from build123d import *

# Parameters (mm, degrees)
SKETCH1_W                    = 295.275
SKETCH1_H                    = 174.625
BASE_FLANGE1_DEPTH           = 3.175
EDGE_FLANGE1_STRIP_W         = 14.1732
EDGE_FLANGE1_STRIP_H         = 3.175
EDGE_FLANGE1_STRIP_CUT_DEPTH = 174.625
EDGE_FLANGE1_DEPTH           = 174.625
EDGE_FLANGE2_STRIP_W         = 14.1732
EDGE_FLANGE2_STRIP_H         = 3.175
EDGE_FLANGE2_STRIP_CUT_DEPTH = 307.2384
EDGE_FLANGE2_DEPTH           = 307.2384
EDGE_FLANGE3_STRIP_W         = 14.1732
EDGE_FLANGE3_STRIP_H         = 3.175
EDGE_FLANGE3_STRIP_CUT_DEPTH = 307.2384
EDGE_FLANGE3_DEPTH           = 307.2384
EDGE_FLANGE4_STRIP_W         = 14.1732
EDGE_FLANGE4_STRIP_H         = 3.175
EDGE_FLANGE4_STRIP_CUT_DEPTH = 166.8018
EDGE_FLANGE4_DEPTH           = 166.8018
EDGE_FLANGE5_STRIP_W         = 14.1732
EDGE_FLANGE5_STRIP_H         = 3.175
EDGE_FLANGE5_STRIP_CUT_DEPTH = 174.625
EDGE_FLANGE5_DEPTH           = 174.625
CUT_EXTRUDE1_REACH           = 437.499
EDGE_FLANGE7_STRIP_W         = 14.1732
EDGE_FLANGE7_STRIP_H         = 3.175
EDGE_FLANGE7_STRIP_CUT_DEPTH = 78.994
EDGE_FLANGE7_DEPTH           = 78.994


# Sheet-metal steps are written as plain solids
with BuildPart() as part:
    # Sketch1 → Base-Flange1 (new body)
    with BuildSketch(Plane(origin=(0, 0, 0), x_dir=(1, 0, 0), z_dir=(0, 1, 0))):
        Rectangle(SKETCH1_W, SKETCH1_H)
    extrude(amount=-BASE_FLANGE1_DEPTH)

    # Edge-Flange1 strip (across the edge) → Edge-Flange1 strip cut (cut)
    with BuildSketch(Plane(origin=(-147.6375, 0, -87.3125), x_dir=(1, 0, 0), z_dir=(0, 0, 1))):
        with Locations((-3.175, -1.5875)):
            Rectangle(EDGE_FLANGE1_STRIP_W, EDGE_FLANGE1_STRIP_H)
    extrude(amount=EDGE_FLANGE1_STRIP_CUT_DEPTH, mode=Mode.SUBTRACT)

    # Edge-Flange1 section (across the edge) → Edge-Flange1 (add)
    with BuildSketch(Plane(origin=(-147.6375, 0, -87.3125), x_dir=(1, 0, 0), z_dir=(0, 0, 1))):
        with BuildLine():
            Line((0, 0.7366), (0, 307.975))
            Line((0, 307.975), (3.175, 307.975))
            Line((3.175, 307.975), (3.175, 0.7366))
            ThreePointArc((3.175, 0.7366), (3.390745145, 0.215745145), (3.9116, 0))
            Line((3.9116, 0), (3.9116, -3.175))
            ThreePointArc((3.9116, -3.175), (1.145681115, -2.029318885), (0, 0.7366))
        make_face()
    extrude(amount=EDGE_FLANGE1_DEPTH)

    # Edge-Flange2 strip (across the edge) → Edge-Flange2 strip cut (cut)
    with BuildSketch(Plane(origin=(-144.4625, 307.975, 87.3125), x_dir=(0, 0, -1), z_dir=(0, -1, 0))):
        with Locations((-3.175, -1.5875)):
            Rectangle(EDGE_FLANGE2_STRIP_W, EDGE_FLANGE2_STRIP_H)
    extrude(amount=EDGE_FLANGE2_STRIP_CUT_DEPTH, mode=Mode.SUBTRACT)

    # Edge-Flange2 section (across the edge) → Edge-Flange2 (add)
    with BuildSketch(Plane(origin=(-144.4625, 307.975, 87.3125), x_dir=(0, 0, -1), z_dir=(0, -1, 0))):
        with BuildLine():
            Line((0, 0.7366), (0, 37.465))
            Line((0, 37.465), (3.175, 37.465))
            Line((3.175, 37.465), (3.175, 0.7366))
            ThreePointArc((3.175, 0.7366), (3.390745145, 0.215745145), (3.9116, 0))
            Line((3.9116, 0), (3.9116, -3.175))
            ThreePointArc((3.9116, -3.175), (1.145681115, -2.029318885), (0, 0.7366))
        make_face()
    extrude(amount=EDGE_FLANGE2_DEPTH)

    # Edge-Flange3 strip (across the edge) → Edge-Flange3 strip cut (cut)
    with BuildSketch(Plane(origin=(-144.4625, 0.7366, -87.3125), x_dir=(0, 0, 1), z_dir=(0, 1, 0))):
        with Locations((-3.175, -1.5875)):
            Rectangle(EDGE_FLANGE3_STRIP_W, EDGE_FLANGE3_STRIP_H)
    extrude(amount=EDGE_FLANGE3_STRIP_CUT_DEPTH, mode=Mode.SUBTRACT)

    # Edge-Flange3 section (across the edge) → Edge-Flange3 (add)
    with BuildSketch(Plane(origin=(-144.4625, 0.7366, -87.3125), x_dir=(0, 0, 1), z_dir=(0, 1, 0))):
        with BuildLine():
            Line((0, 0.7366), (0, 37.465))
            Line((0, 37.465), (3.175, 37.465))
            Line((3.175, 37.465), (3.175, 0.7366))
            ThreePointArc((3.175, 0.7366), (3.390745145, 0.215745145), (3.9116, 0))
            Line((3.9116, 0), (3.9116, -3.175))
            ThreePointArc((3.9116, -3.175), (1.145681115, -2.029318885), (0, 0.7366))
        make_face()
    extrude(amount=EDGE_FLANGE3_DEPTH)

    # Edge-Flange4 strip (across the edge) → Edge-Flange4 strip cut (cut)
    with BuildSketch(Plane(origin=(-144.4625, 307.975, -83.4009), x_dir=(0, -1, 0), z_dir=(0, 0, 1))):
        with Locations((-3.175, -1.5875)):
            Rectangle(EDGE_FLANGE4_STRIP_W, EDGE_FLANGE4_STRIP_H)
    extrude(amount=EDGE_FLANGE4_STRIP_CUT_DEPTH, mode=Mode.SUBTRACT)

    # Edge-Flange4 section (across the edge) → Edge-Flange4 (add)
    with BuildSketch(Plane(origin=(-144.4625, 307.975, -83.4009), x_dir=(0, -1, 0), z_dir=(0, 0, 1))):
        with BuildLine():
            Line((0, 0.7366), (0, 37.465))
            Line((0, 37.465), (3.175, 37.465))
            Line((3.175, 37.465), (3.175, 0.7366))
            ThreePointArc((3.175, 0.7366), (3.390745145, 0.215745145), (3.9116, 0))
            Line((3.9116, 0), (3.9116, -3.175))
            ThreePointArc((3.9116, -3.175), (1.145681115, -2.029318885), (0, 0.7366))
        make_face()
    extrude(amount=EDGE_FLANGE4_DEPTH)

    # Edge-Flange5 strip (across the edge) → Edge-Flange5 strip cut (cut)
    with BuildSketch(Plane(origin=(147.6375, 0, 87.3125), x_dir=(-1, 0, 0), z_dir=(0, 0, -1))):
        with Locations((-3.175, -1.5875)):
            Rectangle(EDGE_FLANGE5_STRIP_W, EDGE_FLANGE5_STRIP_H)
    extrude(amount=EDGE_FLANGE5_STRIP_CUT_DEPTH, mode=Mode.SUBTRACT)

    # Edge-Flange5 section (across the edge) → Edge-Flange5 (add)
    with BuildSketch(Plane(origin=(147.6375, 0, 87.3125), x_dir=(-1, 0, 0), z_dir=(0, 0, -1))):
        with BuildLine():
            Line((0, 0.7366), (0, 307.975))
            Line((0, 307.975), (3.175, 307.975))
            Line((3.175, 307.975), (3.175, 0.7366))
            ThreePointArc((3.175, 0.7366), (3.390745145, 0.215745145), (3.9116, 0))
            Line((3.9116, 0), (3.9116, -3.175))
            ThreePointArc((3.9116, -3.175), (1.145681115, -2.029318885), (0, 0.7366))
        make_face()
    extrude(amount=EDGE_FLANGE5_DEPTH)

    # Sketch29 → Cut-Extrude1 (cut, up to next)
    with BuildSketch(Plane(origin=(147.6375, 0, 0), x_dir=(0, 0, -1), z_dir=(1, 0, 0)), mode=Mode.PRIVATE) as cut_extrude1_sk1:
        Polygon((-87.3125, 37.8968), (-68.5673, 56.642), (-12.3825, 56.642), (8.3185, 77.343), (8.3185, 307.975), (-87.3125, 307.975), align=None)
    cut_extrude1_tool1 = extrude(cut_extrude1_sk1.sketch, amount=-CUT_EXTRUDE1_REACH, mode=Mode.PRIVATE) & part.part
    add(cut_extrude1_tool1.solids().sort_by_distance((147.6375, 182.403147, 40.166664))[0], mode=Mode.SUBTRACT)

    # Edge-Flange7 strip (across the edge) → Edge-Flange7 strip cut (cut)
    with BuildSketch(Plane(origin=(144.4625, 307.975, -8.3185), x_dir=(0, -1, 0), z_dir=(0, 0, -1))):
        with Locations((-3.175, -1.5875)):
            Rectangle(EDGE_FLANGE7_STRIP_W, EDGE_FLANGE7_STRIP_H)
    extrude(amount=EDGE_FLANGE7_STRIP_CUT_DEPTH, mode=Mode.SUBTRACT)

    # Edge-Flange7 section (across the edge) → Edge-Flange7 (add)
    with BuildSketch(Plane(origin=(144.4625, 307.975, -8.3185), x_dir=(0, -1, 0), z_dir=(0, 0, -1))):
        with BuildLine():
            Line((0, 0.7366), (0, 250.19))
            Line((0, 250.19), (3.175, 250.19))
            Line((3.175, 250.19), (3.175, 0.7366))
            ThreePointArc((3.175, 0.7366), (3.390745145, 0.215745145), (3.9116, 0))
            Line((3.9116, 0), (3.9116, -3.175))
            ThreePointArc((3.9116, -3.175), (1.145681115, -2.029318885), (0, 0.7366))
        make_face()
    extrude(amount=EDGE_FLANGE7_DEPTH)


solid = part.part
The listing builds one solid part. Answer for the finished solid, in the listing's coordinates (mm). A direction names the side the tool comes from. Coordinates: 2 decimals unless noted, no trailing zeros. Order: outer loops, then holes, each group sorted by start corner. A loop starts at its lowest first (then second) coordinate and runs counter-clockwise, first axis right, second up. Notation, with made-up numbers: (46.25, 45) -> (61.25, 45) arc R28 ccw to (61.25, 68) -> close; hole circle Ø4 at (72.25, 64). An arc over 180 degrees is marked (long way). Answer in a Markdown table with one row per item. Add a question column.
Item 1: Which of the six approach directions +Z, -Z, +X, -X, +Y, -Y give full straight-line access (tool end or side, diameter ignored) to faces 5 (the face through (-144.462, 155, -1)), 6 (the face through (-2, 0, -1)), 7 (the face through (146.07, 47.14, 78.07))?
Item 2: Find section A-A (x = -50). Write down the section's boundary in (y, z) (1 decimal).
Item 3: Find section B-B (x = -111.5). Write down the section's boundary in (y, z) (1 decimal), then the cut area to 4 significant figures.
Item 4: Find section D-D (z = -30). Write down the section's boundary in (x, y) (1 decimal), then the cut area to 3 significant figures.
Item 5: Determine the mould class of faces 1 (the face through (-2, -3.175, -1)), 2 (the face through (-125, 152, -84.138)), 3 (the face through (17, 304.8, -47)), 4 (the face through (-126, 307.975, -1)) for opening direction Y: +Y half, -Y half, draft (parallel to the pull), parting line (faces both ways), or undercut.
Item 6: Find the intervals of material crossed by L1, parallel to X at y = 79, z = -60; L2, parallel to Y at x = -130, z = -36.5 (3 decimals); L3, parallel to X at y = 264, z = 67, in increasing order. Write a range as from..to.
Item 7: Each of these flat-tipped pins is pushed along its axis until it touches: P1, Ø3.5, axis at y = 306.5, z = -38, coming from the -X side; P2, Ø1, axis at x = -145.5, y = 305.5, coming from the +Z side; P3, Ø10, axis at y = 276.5, z = 53, coming from the +X side. Where does it stop, or does it pass through?
Item 8: Find section C-C (y = 281.5). Write down the section's boundary in (x, z), then the cut area to 3 significant figures.
Result set:
| question | item | result |
|---|---|---|
| 1 | face 5 | none |
| 1 | face 6 | +Z, -Z |
| 1 | face 7 | +Z, +X, +Y |
| 2 | outline | (-3.2, -87.3) -> (0, -87.3) -> (0, 87.3) -> (-3.2, 87.3) -> close; (304.8, -87.3) -> (308, -87.3) -> (308, -8.3) -> (304.8, -8.3) -> close |
| 3 | outline | (-3.2, -87.3) -> (0, -87.3) -> (0, 87.3) -> (-3.2, 87.3) -> close; (0.7, -87.3) -> (308, -87.3) -> (308, -84.1) -> (0.7, -84.1) -> close; (0.7, 84.1) -> (308, 84.1) -> (308, 87.3) -> (0.7, 87.3) -> close; (304.8, -83.4) -> (308, -83.4) -> (308, 83.4) -> (304.8, 83.4) -> close |
| 3 | area | 3,035 mm² |
| 4 | outline | (-147.6, 0.7) arc R3.9 ccw to (-143.7, -3.2) -> (143.7, -3.2) arc R3.9 ccw to (147.6, 0.7) -> (147.6, 304.1) arc R3.9 ccw to (143.7, 308) -> (-105.7, 308) -> (-105.7, 304.8) -> (143.7, 304.8) arc R0.7 cw to (144.5, 304.1) -> (144.5, 0.7) arc R0.7 cw to (143.7, 0) -> (-143.7, 0) arc R0.7 cw to (-144.5, 0.7) -> (-144.5, 304.1) arc R0.7 cw to (-143.7, 304.8) -> (-107, 304.8) -> (-107, 308) -> (-143.7, 308) arc R3.9 ccw to (-147.6, 304.1) -> close |
| 4 | area | 3,790 mm² |
| 5 | face 1 | -Y half |
| 5 | face 2 | draft |
| 5 | face 3 | undercut |
| 5 | face 4 | +Y half |
| 6 | L1 | x = -147.64..-144.46, 144.46..147.64 |
| 6 | L2 | y = -3.175..0, 304.8..307.975 |
| 6 | L3 | x = -147.64..-144.46 |
| 7 | P1 | stops at x = -147.58 |
| 7 | P2 | stops at z = 87.1 |
| 7 | P3 | stops at x = -144.46 |
| 8 | outline | (-147.64, -83.4) arc R3.91 ccw to (-143.73, -87.31) -> (-107, -87.31) -> (-107, -84.14) -> (-143.73, -84.14) arc R0.74 cw to (-144.46, -83.4) -> (-144.46, 83.4) arc R0.74 cw to (-143.73, 84.14) -> (-107, 84.14) -> (-107, 87.31) -> (-143.73, 87.31) arc R3.91 ccw to (-147.64, 83.4) -> close; (144.46, -87.31) -> (147.64, -87.31) -> (147.64, -8.32) -> (144.46, -8.32) -> close |
| 8 | area | 1,040 mm² |
